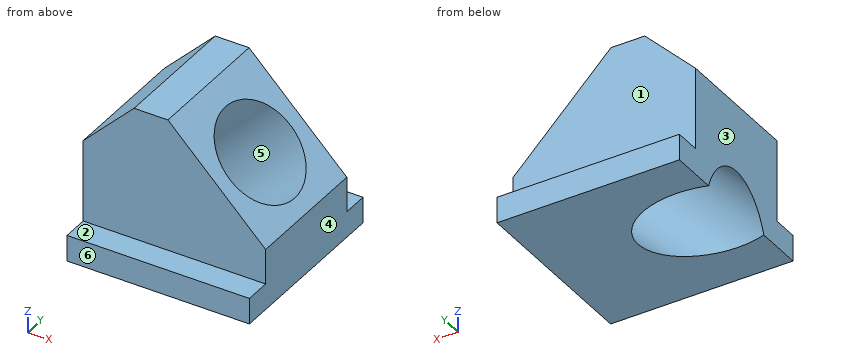
```python
from build123d import *

# Parameters (mm, degrees)
F0_W     = 71.12
F0_H     = 71.12
F1_DEPTH = 10.16
F2_W     = 71.12
F2_H     = 50.8
F3_DEPTH = 51.816
F5_DEPTH = 71.12
F7_DEPTH = 71.12
F8_R     = 19.05
F9_DEPTH = 101.6


with BuildPart() as f1:
    # F0 (on Top) → F1 (new body)
    with BuildSketch(Plane.XY):
        with Locations((17.602327, -4.579058)):
            Rectangle(F0_W, F0_H)
    extrude(amount=F1_DEPTH)

    # F2 (on face) → F3 (join)
    with BuildSketch(Plane.XY.offset(10.16)):
        with Locations((17.602327, -4.579058)):
            Rectangle(F2_W, F2_H)
    extrude(amount=F3_DEPTH)

    # F4 (on face) → F5 (cut)
    with BuildSketch(Plane.XZ.offset(29.979058)):
        Polygon((-17.957673, 61.976), (-17.957673, 42.149723), (1.868605, 61.976), align=None)
    extrude(amount=-F5_DEPTH, mode=Mode.SUBTRACT)

    # F6 (on face) → F7 (cut)
    with BuildSketch(Plane.XZ.offset(29.979058)):
        Polygon((15.062327, 61.976), (53.162327, 23.876), (53.162327, 61.976), align=None)
    extrude(amount=-F7_DEPTH, mode=Mode.SUBTRACT)

    # F8 (on face) → F9 (cut)
    with BuildSketch(Plane(origin=(38.519164, 0, 38.519164), x_dir=(0.707107, 0, -0.707107), z_dir=(0.707107, 0, 0.707107))):
        with Locations((-4.691439, -4.579058)):
            Circle(F8_R)
    extrude(amount=-F9_DEPTH, mode=Mode.SUBTRACT)


solid = f1.part
```
Could you check a few things on this model? Use its own coordinates, in mm. Face numbers are marked on the shaded views. A direction names the side the tool comes from. Round coordinates to 2 decimals unless told otherwise and drop trailing zeros. Order: outer loops, then holes, each group sorted by start corner. A loop starts at its lowest first (then second) coordinate and runs counter-clockwise, first axis right, second up. Notation, with made-up numbers: (67.5, -6.75) -> (94.5, -6.75) arc R23 ccw to (94.5, 8.25) -> close; hole circle Ø3 at (-35.5, 57.5). An arc over 180 degrees is marked (long way). One line per question, with ' | ' between items.
Q1. Which directions (+Z, -Z, +X, -X, +Y, -Y) give clear straight access to the entire face, cutting with the end or side of a thin tool? Please do the marked faces 1, 2 and 3.
Computed values:
face 1: +Z, +X, -X, +Y | face 2: +Z, +X, -X, -Y | face 3: +Z, -Z, -X, +Y, -Y
Q2. If we section it at A-A on y = 9.5: Write out the boundary of the cut face in (x, z), plus the area to 3 significant figures.
Computed values:
outline: (-17.96, 6.83) -> (26.13, 50.91) -> (15.06, 61.98) -> (1.87, 61.98) -> (-17.96, 42.15) -> close; (11.51, 0) -> (53.16, 0) -> (53.16, 23.88) -> (44.28, 32.76) -> close | area: 1,990 mm²
Q3. If I drill on line 1 (Y direction, x = 22, z = 43); line 2 (Z direction, x = 13, y = 25); line 3 (Y direction, x = -3.5, z = 55), over which ranges is the centre line in solid material (lowest first)? Write a range as from..to.
Computed values:
line 1: -29.98..-20.69, 11.54..20.82 | line 2: 0..10.16 | line 3: -29.98..20.82
Q4. If we section it at B-B on y = 17.5: Write out the boundary of the cut face in (x, z), plus the area to 3 significant figures.
Computed values:
outline: (-17.96, 0) -> (53.16, 0) -> (53.16, 23.88) -> (15.06, 61.98) -> (1.87, 61.98) -> (-17.96, 42.15) -> close | area: 3,490 mm²
Q5. If we section it at C-C on y = -2: Write out the boundary of the cut face in (x, z).
Computed values:
outline: (-17.96, 15.37) -> (21.86, 55.18) -> (15.06, 61.98) -> (1.87, 61.98) -> (-17.96, 42.15) -> close; (20.06, 0) -> (53.16, 0) -> (53.16, 23.88) -> (48.55, 28.49) -> close
Q6. If we section it at D-D on z = 57: Write out the boundary of the cut face in (x, y), plus the area to 3 significant figures.
Computed values:
outline: (-3.11, -29.98) -> (20.04, -29.98) -> (20.04, 20.82) -> (-3.11, 20.82) -> close | area: 1,180 mm²
Q7. We'd pull the mould along X, two halves only. Please class the marked faces 4, 5 and 6: released by +X, released by -X, zero draft, split by the parting line, or undercut.
Computed values:
face 4: released by +X | face 5: undercut | face 6: zero draft
Q8. I'm going to push flat-ended pins straight in: pin 1 (3 mm diameter, centred on x = 25, y = 25.5, fed in from +Z); pin 2 (2 mm diameter, centred on y = 17.5, z = 42, fed in from +X); pin 3 (1 mm diameter, centred on y = -9.5, z = 40, fed in from +X). Where does each tip first touch, or does it pass through?
Computed values:
pin 1: z = 10.16 | pin 2: x = 36.04 | pin 3: x = 7.87
